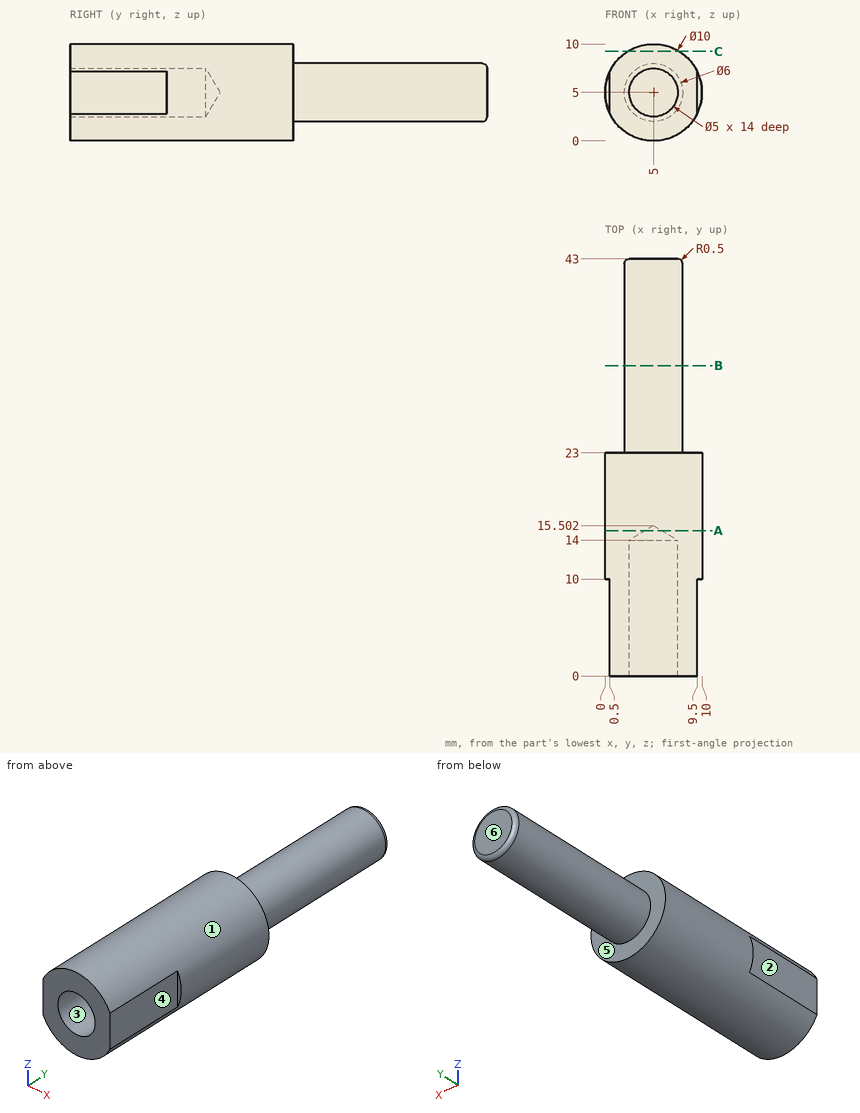
Source: three-view drawing plus pictorial views. Frame: mm from the lowest corner of the part. A direction names the side the tool comes from. Coordinates: 2 decimals unless noted, no trailing zeros. Loops run counter-clockwise (first coordinate to the right, second up) from the corner with the lowest first, then second, coordinate; pieces in that order, holes last. Notation, with made-up numbers: M -6.75,-27 L 11.25,-27 A28 cw 11.25,2 Z; hole C 21,28.25 d3. An arc over 180 degrees is marked long. Use CSV: the item, a comma, the result in double quotes.
(1) Reachability of the marked faces 4, 5 and 6 from +Z, -Z, +X, -X, +Y, -Y: full face, straight path, thin tool, end or side. Return the list, or none.
Answers follow:
face 4,"+Z, -Z, +X, -Y"
face 5,"+Y"
face 6,"+Z, -Z, +X, -X, +Y"
(2) Contact query for flat-ended pins moving along their axis: pin 1 (2 mm diameter, centred on y = 7.5, z = 4, fed in from +X); pin 2 (5 mm diameter, centred on y = 27, z = 4, fed in from +X); pin 3 (1.5 mm diameter, centred on y = 19, z = 8.5, fed in from +X). Output: stop coordinate, or through.
Answers follow:
pin 1,"x = 9.5"
pin 2,"x = 8"
pin 3,"x = 9.18"
(3) Cut plane A-A on y = 15. Return loops of the section in (x, z).
Answers follow:
outline,"C 5,5 d10; hole C 5,5 d1.67"
(4) Line query: line 1 (Z direction, x = 5, y = 5.25); line 2 (X direction, y = 7, z = 5); line 3 (Y direction, x = 7.25, z = 2). Output: solid intervals per line, ascending. Write a range as [from, to].
Answers follow:
line 1,"[0, 2.5], [7.5, 10]"
line 2,"[0.5, 2.5], [7.5, 9.5]"
line 3,"[0, 23]"
(5) Draft query along X for the marked faces 1, 2 and 3. Return one class per face: pulls with the +X half, pulls with the -X half, needs draft (parallel to the pull), parting line crosses it, or undercut.
Answers follow:
face 1,"parting line crosses it"
face 2,"pulls with the -X half"
face 3,"undercut"
(6) Cut plane C-C on z = 9.25. Return loops of the section in (x, y).
Answers follow:
outline,"M 2.37,0 L 7.63,0 L 7.63,23 L 2.37,23 Z"
(7) Cut plane B-B on y = 32. Return loops of the section in (x, z), and give its area (3 significant figures).
Answers follow:
outline,"C 5,5 d6"
area,"28.3 mm²"
